For this review, take the finished solid that the model builds, in its own axes (mm). Round coordinates to 2 decimals unless told otherwise and drop trailing zeros. Write each loop counter-clockwise with the first axis right and the second up, starting at its lowest first coordinate (ties: lowest second). Pieces come first, ordered by that corner, then holes. Notation, with made-up numbers: M 88.25,48.25 L 108.25,48.25 A17 cw 108.25,70.25 Z; hole C -30.5,22.5 d11. An arc over 180 degrees is marked long. Write each question's results on one line, items separated by ' | '. Start each with the question number.
```python
from build123d import *

# Parameters (mm, degrees)
CORTAR_EXTRUIR1_START      = -50
CROQUIS2_R                 = 4.324629937
CORTAR_EXTRUIR1_DEPTH      = 25
CROQUIS3_W                 = 1202
CROQUIS3_H                 = 602
SALIENTE_EXTRUIR1_DEPTH    = 31
CROQUIS4_W                 = 40
CROQUIS4_H                 = 40
SALIENTE_EXTRUIR2_DEPTH    = 750
CORTAR_EXTRUIR2_DEPTH      = 1031.418846877
CORTAR_EXTRUIR2_DEPTH_BACK = 1031.418846877
CROQUIS5_W                 = 169.23973075
CROQUIS5_H                 = 94.141610947


with BuildPart() as part:
    # Croquis1 → Revolución1 (revolve)
    with BuildSketch(Plane.XY, mode=Mode.PRIVATE) as revoluci_n1_sk:
        Polygon((0, 0), (0, 80), (-58, 80), (-58, 31.455108359), (-67.5, 0), align=None)
    revolve(revoluci_n1_sk.sketch.rotate(Axis((0, 0, 0), (0, 1, 0)), 180), axis=Axis((0, 0, 0), (0, 1, 0)))

    # Croquis2 → Cortar-Extruir1 (cut)
    with BuildSketch(Plane(origin=(0, 80, 0), x_dir=(1, 0, 0), z_dir=(0, 1, 0)).offset(CORTAR_EXTRUIR1_START)):
        with Locations((0, 63.025248345)):
            Circle(CROQUIS2_R)
        with Locations((63.025248345, 0)):
            Circle(CROQUIS2_R)
        with Locations((0, -63.025248345)):
            Circle(CROQUIS2_R)
        with Locations((-63.025248345, 0)):
            Circle(CROQUIS2_R)
    extrude(amount=-CORTAR_EXTRUIR1_DEPTH, mode=Mode.SUBTRACT)

    # Croquis3 → Saliente-Extruir1 (add)
    with BuildSketch(Plane.XZ):
        Rectangle(CROQUIS3_W, CROQUIS3_H)
    extrude(amount=SALIENTE_EXTRUIR1_DEPTH)

    # Croquis4 → Saliente-Extruir2 (add)
    with BuildSketch(Plane.XZ.offset(31)):
        with Locations((-551, 251)):
            Rectangle(CROQUIS4_W, CROQUIS4_H)
        with Locations((559, 251)):
            Rectangle(CROQUIS4_W, CROQUIS4_H)
        with Locations((559, -249)):
            Rectangle(CROQUIS4_W, CROQUIS4_H)
        with Locations((-551, -249)):
            Rectangle(CROQUIS4_W, CROQUIS4_H)
    extrude(amount=SALIENTE_EXTRUIR2_DEPTH)

    # Croquis5 → Cortar-Extruir2 (cut, two sides: drawn at the far end of the back side and taken through both)
    with BuildSketch(Plane.XY.offset(-CORTAR_EXTRUIR2_DEPTH_BACK)):
        with Locations((-9.450479153, 47.070805474)):
            Rectangle(CROQUIS5_W, CROQUIS5_H)
    extrude(amount=CORTAR_EXTRUIR2_DEPTH + CORTAR_EXTRUIR2_DEPTH_BACK, mode=Mode.SUBTRACT)


solid = part.part
```
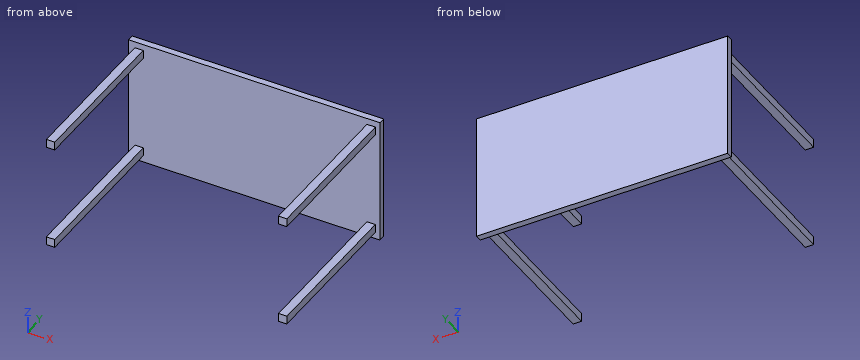
Item 1: We need section B-B on z = 1. State the section outline as (x, y) points, then the cut area to 3 significant figures.
Item 2: For probe 1 along Y at (x, z) = (543.5, 105), list the stretches that pass through material, from the lowest coordinate up.
Item 3: We need section C-C on x = 280. State the section outline as (y, z) points, then the cut area to 3 significant figures.
Item 4: Insertion check: P1, Ø20, axis at y = -562.5, z = -258.5, coming from the -X side; P2, Ø20, axis at x = 565, y = -501.5, coming from the -Z side; P3, Ø1, axis at x = -204.5, z = -234.5, coming from the +Y side; P4, Ø12, axis at x = 567, y = -245, coming from the +Z side. Each pin has a flat end and moves straight along its axis. Give the tip position at first contact, or say it passes through.
Item 5: We need section A-A on y = -635. State the section outline as (x, z) points, then the cut area to 3 significant figures.
Numbers:
1) outline: M -601,-31 L 601,-31 L 601,0 L -601,0 Z | area: 37,300 mm^2
2) probe 1: y = -31 to 0
3) outline: M -31,-301 L 0,-301 L 0,301 L -31,301 Z | area: 18,700 mm^2
4) P1: stops at x = -571 | P2: stops at z = -269 | P3: stops at y = 0 | P4: stops at z = 271
5) outline: M -571,-269 L -531,-269 L -531,-229 L -571,-229 Z; M -571,231 L -531,231 L -531,271 L -571,271 Z; M 539,-269 L 579,-269 L 579,-229 L 539,-229 Z; M 539,231 L 579,231 L 579,271 L 539,271 Z | area: 6,400 mm^2
